Here's how the part is built. I have some questions about the finished solid (model axes, mm). A direction names the side the tool comes from. Round coordinates to 2 decimals unless told otherwise and drop trailing zeros. Order: outer loops, then holes, each group sorted by start corner. A loop starts at its lowest first (then second) coordinate and runs counter-clockwise, first axis right, second up. Notation, with made-up numbers: M 38.25,-36 L 55.25,-36 A24 ccw 55.25,-23 Z; hole C 39.5,55.25 d4. An arc over 180 degrees is marked long. Write item = value, one per line. Start each with the question number.
Item 1: I want a section at D-D, the plane x = 28. List the corners of the cut face in (y, z) for me, plus the area to 3 significant figures.
Item 2: I want a section at A-A, the plane x = 80. List the corners of the cut face in (y, z) for me, plus the area to 3 significant figures.
Item 3: I want a section at B-B, the plane y = -60.5. List the corners of the cut face in (x, z) for me (1 decimal), plus the area to 3 significant figures.
Item 4: We'd pull the mould along Y, two halves only. Please class faces 1 (the face through (55, -77, 4.325)), 2 (the face through (36.38, -76.14, 1.41)), 3 (the face through (98.193, -56.237, 0.022)), 4 (the face through (34, -80.2, 9)): pulls with the +Y half, pulls with the -Y half, needs draft (parallel to the pull), parting line crosses it, or undercut.
Item 5: I want a section at C-C, the plane z = 10. List the corners of the cut face in (x, y) for me, plus the area to 3 significant figures.
Item 6: I'm going to push flat-ended pins straight in: P1, Ø12, axis at x = 30, y = -73, coming from the +Z side; P2, Ø8, axis at x = 51, y = -74, coming from the -Z side; P3, Ø8.5, axis at x = 28, z = 4, coming from the -Y side; P4, Ø2, axis at x = 43, z = 12, coming from the +Y side. Where does each tip first touch, or does it pass through?
Item 7: For faces 5 (the face through (17, -76, 11.825)), 6 (the face through (95, -95, 1.588)), 7 (the face through (35.943, -76.144, 11.302)), which set-ups out of +Z, -Z, +X, -X, +Y, -Y let a thin tool reach every point of the face, with its end or its side?
Item 8: Please list where these lines run through material, in increasing order: L1, parallel to Z at x = 92.5, y = -57 (1 decimal); L2, parallel to Y at x = 85, z = 0.75; L3, parallel to Y at x = 77, z = 3.
```python
from build123d import *

# Parameters (mm, degrees)
SKETCH2_R           = 4
BOSS_EXTRUDE1_DEPTH = 1.5875
BOSS_EXTRUDE2_START = 15
SKETCH2_3_R         = 4
BOSS_EXTRUDE2_DEPTH = 3.175
BOSS_EXTRUDE3_START = 7.5
SKETCH2_5_R         = 4
BOSS_EXTRUDE3_DEPTH = 3.175
SKETCH3_W           = 4
SKETCH3_H           = 3.175
BOSS_EXTRUDE5_DEPTH = 4
SKETCH5_W           = 4
SKETCH5_H           = 3.175
BOSS_EXTRUDE6_DEPTH = 4
SKETCH7_W           = 4
SKETCH7_H           = 3.175
BOSS_EXTRUDE8_DEPTH = 4


with BuildPart() as part:
    # Sketch2 → Boss-Extrude1 (new, symmetric)
    with BuildSketch(Plane.XY):
        with Locations((16.7, -76.2)):
            Circle(SKETCH2_R)
        with Locations((94.5382, -57.8618)):
            Circle(SKETCH2_R)
        with Locations((94.5382, -94.5382)):
            Circle(SKETCH2_R)
        with BuildLine():
            ThreePointArc((20.7, -76.2), (19.528427125, -73.371572875), (16.7, -72.2))
            Line((16.7, -72.2), (16.7, -80.2))
            ThreePointArc((16.7, -80.2), (19.528427125, -79.028427125), (20.7, -76.2))
        make_face()
        with BuildLine():
            Line((16.7, -80.2), (16.7, -72.2))
            ThreePointArc((16.7, -72.2), (12.7, -76.2), (16.7, -80.2))
        make_face()
        with BuildLine():
            ThreePointArc((98.5382, -57.8618), (96.68064547, -54.483941594), (92.833236295, -54.243361281))
            Line((92.833236295, -54.243361281), (96.243163705, -61.480238719))
            ThreePointArc((96.243163705, -61.480238719), (97.916058406, -60.00424547), (98.5382, -57.8618))
        make_face()
        with BuildLine():
            Line((96.243163705, -61.480238719), (92.833236295, -54.243361281))
            ThreePointArc((92.833236295, -54.243361281), (90.919761281, -59.566763705), (96.243163705, -61.480238719))
        make_face()
        with BuildLine():
            ThreePointArc((96.243163705, -90.919761281), (90.919761281, -92.833236295), (92.833236295, -98.156638719))
            Line((92.833236295, -98.156638719), (96.243163705, -90.919761281))
        make_face()
        with BuildLine():
            Line((96.243163705, -90.919761281), (92.833236295, -98.156638719))
            ThreePointArc((92.833236295, -98.156638719), (96.68064547, -97.916058406), (98.5382, -94.5382))
            ThreePointArc((98.5382, -94.5382), (97.916058406, -92.39575453), (96.243163705, -90.919761281))
        make_face()
    extrude(amount=BOSS_EXTRUDE1_DEPTH, both=True)



with BuildPart() as body_2:
    # Sketch2_3 → Boss-Extrude2 (new body)
    with BuildSketch(Plane.XY.offset(BOSS_EXTRUDE2_START)):
        with Locations((94.5382, -57.8618)):
            Circle(SKETCH2_3_R)
        with Locations((94.5382, -94.5382)):
            Circle(SKETCH2_3_R)
        with Locations((16.7, -76.2)):
            Circle(SKETCH2_3_R)
        with BuildLine():
            ThreePointArc((20.7, -76.2), (19.528427125, -73.371572875), (16.7, -72.2))
            Line((16.7, -72.2), (16.7, -80.2))
            ThreePointArc((16.7, -80.2), (19.528427125, -79.028427125), (20.7, -76.2))
        make_face()
        with BuildLine():
            Line((16.7, -80.2), (16.7, -72.2))
            ThreePointArc((16.7, -72.2), (12.7, -76.2), (16.7, -80.2))
        make_face()
        with BuildLine():
            ThreePointArc((98.5382, -57.8618), (96.68064547, -54.483941594), (92.833236295, -54.243361281))
            Line((92.833236295, -54.243361281), (96.243163705, -61.480238719))
            ThreePointArc((96.243163705, -61.480238719), (97.916058406, -60.00424547), (98.5382, -57.8618))
        make_face()
        with BuildLine():
            Line((96.243163705, -61.480238719), (92.833236295, -54.243361281))
            ThreePointArc((92.833236295, -54.243361281), (90.919761281, -59.566763705), (96.243163705, -61.480238719))
        make_face()
        with BuildLine():
            ThreePointArc((96.243163705, -90.919761281), (90.919761281, -92.833236295), (92.833236295, -98.156638719))
            Line((92.833236295, -98.156638719), (96.243163705, -90.919761281))
        make_face()
        with BuildLine():
            Line((96.243163705, -90.919761281), (92.833236295, -98.156638719))
            ThreePointArc((92.833236295, -98.156638719), (96.68064547, -97.916058406), (98.5382, -94.5382))
            ThreePointArc((98.5382, -94.5382), (97.916058406, -92.39575453), (96.243163705, -90.919761281))
        make_face()
    extrude(amount=-BOSS_EXTRUDE2_DEPTH)


with BuildPart() as body_3:
    # Sketch2_5 → Boss-Extrude3 (new body)
    with BuildSketch(Plane.XY.offset(BOSS_EXTRUDE3_START)):
        with Locations((55.6191, -76.2)):
            Circle(SKETCH2_5_R)
        with BuildLine():
            ThreePointArc((55.6191, -72.2), (54.745531135, -72.296555695), (53.914136295, -72.581561281))
            Line((53.914136295, -72.581561281), (55.6191, -76.2))
            Line((55.6191, -76.2), (55.6191, -72.2))
        make_face()
        with BuildLine():
            Line((57.324063705, -79.818438719), (55.6191, -76.2))
            Line((55.6191, -76.2), (55.6191, -80.2))
            ThreePointArc((55.6191, -80.2), (56.492668865, -80.103444305), (57.324063705, -79.818438719))
        make_face()
        with BuildLine():
            Line((55.6191, -72.2), (55.6191, -76.2))
            Line((55.6191, -76.2), (57.324063705, -72.581561281))
            ThreePointArc((57.324063705, -72.581561281), (56.492668865, -72.296555695), (55.6191, -72.2))
        make_face()
        with BuildLine():
            Line((55.6191, -80.2), (55.6191, -76.2))
            Line((55.6191, -76.2), (53.914136295, -79.818438719))
            ThreePointArc((53.914136295, -79.818438719), (54.745531135, -80.103444305), (55.6191, -80.2))
        make_face()
        with BuildLine():
            Line((55.6191, -76.2), (53.914136295, -72.581561281))
            ThreePointArc((53.914136295, -72.581561281), (51.6191, -76.2), (53.914136295, -79.818438719))
            Line((53.914136295, -79.818438719), (55.6191, -76.2))
        make_face()
        with BuildLine():
            Line((57.324063705, -72.581561281), (55.6191, -76.2))
            Line((55.6191, -76.2), (57.324063705, -79.818438719))
            ThreePointArc((57.324063705, -79.818438719), (58.996958406, -78.34244547), (59.6191, -76.2))
            ThreePointArc((59.6191, -76.2), (58.996958406, -74.05755453), (57.324063705, -72.581561281))
        make_face()
    extrude(amount=-BOSS_EXTRUDE3_DEPTH)


with BuildPart() as part_1:
    add(part.part)

    add(body_2.part)  # Boss-Extrude5 merges body 2

    add(body_3.part)  # Boss-Extrude5 merges body 3
    # Sketch3 → Boss-Extrude5 (add, symmetric)
    with BuildSketch(Plane(origin=(0, -76.2, 0), x_dir=(1, 0, 0), z_dir=(0, 1, 0))):
        with Locations((53.6191, -5.9125)):
            Rectangle(SKETCH3_W, SKETCH3_H)
        Polygon((51.6191, -7.5), (44.299946785, -6.100396086), (20.7, -11.825), (20.7, -15), align=None)
        Polygon((51.6191, -7.5), (51.6191, -4.325), (44.299946785, -6.100396086), align=None)
        Polygon((51.6191, -4.325), (20.7, 1.5875), (20.7, -1.5875), (44.299946785, -6.100396086), align=None)
        with Locations((18.7, 0)):
            Rectangle(SKETCH3_W, SKETCH3_H)
        with Locations((18.7, -13.4125)):
            Rectangle(SKETCH3_W, SKETCH3_H)
    extrude(amount=BOSS_EXTRUDE5_DEPTH, both=True)

    # Sketch5 → Boss-Extrude6 (add, symmetric)
    with BuildSketch(Plane(origin=(-19.276371181, -40.910177532, 0), x_dir=(-0.9046096798275906, 0.4262409261934197, 0), z_dir=(-0.42624092619341963, -0.9046096798275904, 0))):
        with Locations((-84.793134819, -5.9125)):
            Rectangle(SKETCH5_W, SKETCH5_H)
        Polygon((-86.793134819, -7.5), (-86.793134819, -4.325), (-95.083781445, -6.100396086), align=None)
        Polygon((-86.793134819, -4.325), (-121.816220762, 1.5875), (-121.816220762, -1.5875), (-95.083781445, -6.100396086), align=None)
        Polygon((-86.793134819, -7.5), (-95.083781445, -6.100396086), (-121.816220762, -11.825), (-121.816220762, -15), align=None)
        with Locations((-123.816220762, 0)):
            Rectangle(SKETCH5_W, SKETCH5_H)
        with Locations((-123.816220762, -13.4125)):
            Rectangle(SKETCH5_W, SKETCH5_H)
    extrude(amount=BOSS_EXTRUDE6_DEPTH, both=True)

    # Sketch7 → Boss-Extrude8 (add, symmetric)
    with BuildSketch(Plane(origin=(39.486274988, -83.801588208, 0), x_dir=(0.9046096798275907, 0.4262409261934195, 0), z_dir=(-0.4262409261934195, 0.9046096798275907, 0))):
        with Locations((19.834017667, -5.9125)):
            Rectangle(SKETCH7_W, SKETCH7_H)
        Polygon((30.124664293, -6.100396086), (21.834017667, -4.325), (21.834017667, -7.5), align=None)
        Polygon((56.85710361, -1.5875), (56.85710361, 1.5875), (21.834017667, -4.325), (30.124664293, -6.100396086), align=None)
        with Locations((58.85710361, 0)):
            Rectangle(SKETCH7_W, SKETCH7_H)
        Polygon((30.124664293, -6.100396086), (21.834017667, -7.5), (56.85710361, -15), (56.85710361, -11.825), align=None)
        with Locations((58.85710361, -13.4125)):
            Rectangle(SKETCH7_W, SKETCH7_H)
    extrude(amount=BOSS_EXTRUDE8_DEPTH, both=True)


solid = part_1.part
```
Filled in:
q1.outline = M -80.2,-0.19 L -72.2,-0.19 L -72.2,2.98 L -80.2,2.98 Z; M -80.2,10.05 L -72.2,10.05 L -72.2,13.23 L -80.2,13.23 Z
q1.area = 50.8 mm^2
q2.outline = M -92.11,0.13 L -83.27,0.77 L -83.27,3.94 L -92.11,3.31 Z; M -92.11,9.64 L -83.27,8.84 L -83.27,12.01 L -92.11,12.82 Z; M -69.13,0.77 L -60.29,0.13 L -60.29,3.31 L -69.13,3.94 Z; M -69.13,8.84 L -60.29,9.64 L -60.29,12.82 L -69.13,12.01 Z
q2.area = 112 mm^2
q3.outline = M 79.6,0.2 L 91.4,-1.6 L 97.5,-1.6 L 97.5,1.6 L 91.4,1.6 L 79.6,3.4 Z; M 79.6,9.5 L 91.4,11.8 L 97.5,11.8 L 97.5,15 L 91.4,15 L 79.6,12.7 Z
q3.area = 114 mm^2
q4.face_1 = undercut
q4.face_2 = needs draft
q4.face_3 = undercut
q4.face_4 = pulls with the -Y half
q5.outline = M 28.22,-80.2 L 41.31,-80.2 L 41.31,-72.2 L 28.22,-72.2 Z; M 68.09,-86.5 L 81.51,-92.82 L 84.92,-85.58 L 71.5,-79.26 Z; M 68.09,-65.9 L 71.5,-73.14 L 84.92,-66.82 L 81.51,-59.58 Z
q5.area = 342 mm^2
q6.P1 = 14.2
q6.P2 = 3.44
q6.P3 = -80.2
q6.P4 = through
q7.face_5 = -X, +Y, -Y
q7.face_6 = +X, -Y
q7.face_7 = +Z, +Y, -Y
q8.L1 = -1.6 to 1.6, 11.8 to 15
q8.L2 = -94.47 to -85.62, -66.78 to -57.93
q8.L3 = -90.7 to -81.85, -70.55 to -61.7
